The model under review builds one solid part; all positions refer to its coordinate system, in mm. Face numbers are marked on the shaded views. A direction names the side the tool comes from. Round coordinates to 2 decimals unless told otherwise and drop trailing zeros. Order: outer loops, then holes, each group sorted by start corner. A loop starts at its lowest first (then second) coordinate and runs counter-clockwise, first axis right, second up. Notation, with made-up numbers: M 62,9.5 L 112,9.5 A38 ccw 112,48.5 Z; hole C -30,29.5 d5. An arc over 180 degrees is marked long. Answer as a JSON object with one key per item and string values. Group by question number.
1. Add section B-B on z = 23. State the section outline as (x, y) points, and give its area (3 significant figures).
2. To check wall thickness, follow probe 1 along X at (y, z) = (-7.5, 8.25); probe 2 along Z at (x, y) = (15.5, 2); probe 3 along Y at (x, z) = (38, 5). State the ranges of each line that lie inside material, in increasing order. Write a range as [from, to].
3. Add section D-D on z = 5.5. State the section outline as (x, y) points.
4. Clearance check with flat-ended pins moving along their axes: P1, Ø4, axis at x = 23, z = 15.5, coming from the +Y side; P2, Ø1, axis at x = 22.5, z = 8.5, coming from the -Y side; P3, Ø8, axis at x = 26, z = 16, coming from the +Y side. State where each tip first meets the part, or that it passes through.
5. Add section A-A on y = -37. State the section outline as (x, z) points.
6. Mouldability with a two-part tool opening along X and no side actions: class the marked faces 4, 5 and 6 as released by +X, released by -X, zero draft, split by the parting line, or undercut.
7. Add section C-C on y = -13.5. State the section outline as (x, z) points.
8. Machinability: for the marked faces 1, 2 and 3, which of the approach directions +Z, -Z, +X, -X, +Y, -Y give a long, thin tool a straight path to every point of the face, cutting with its end or side? Answer none if there is none.
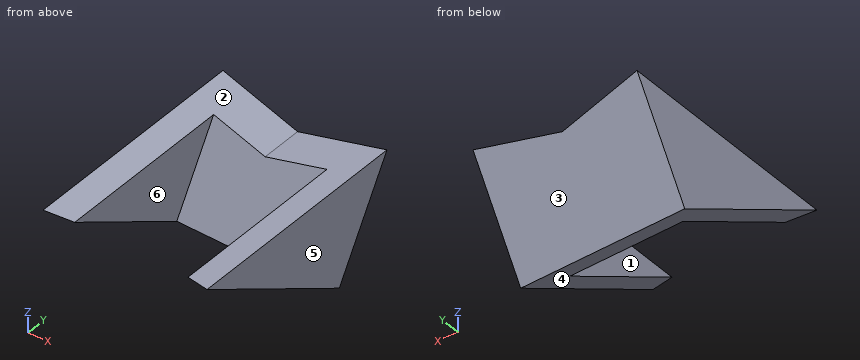
```python
from build123d import *

# Parameters (mm, degrees)
EXTRUDE_1_DEPTH     = 42
CUT_EXTRUDE_3_DEPTH = 77.352761936
SKETCH_4_W          = 29
SKETCH_4_H          = 38.596109301
CUT_EXTRUDE_4_DEPTH = 42


with BuildPart() as part:
    # Эскиз1 → Бобышка-Вытянуть1 (new body)
    with BuildSketch(Plane(origin=(0, 0, 0), x_dir=(0, 0, -1), z_dir=(1, 0, 0))):
        Polygon((0, 0), (-25.751903746, 15.473304826), (-25.751903746, -42.858365035), align=None)
    extrude(amount=EXTRUDE_1_DEPTH)

    # Эскиз3 → Вырез-Вытянуть3 (cut, through all)
    with BuildSketch(Plane(origin=(0, 15.473304826, 0), x_dir=(1, 0, 0), z_dir=(0, 1, 0))):
        Polygon((0, -25.751903746), (21, -21.751903746), (42, -25.751903746), align=None)
    extrude(amount=-CUT_EXTRUDE_3_DEPTH, mode=Mode.SUBTRACT)

    # Эскиз4 → Вырез-Вытянуть4 (cut)
    with BuildSketch(Plane(origin=(0, 0, 0), x_dir=(-1, 0, 0), z_dir=(0, -0.5150380749100486, -0.8571673007021157))):
        with Locations((-21, -28.298054651)):
            Rectangle(SKETCH_4_W, SKETCH_4_H)
    extrude(amount=-CUT_EXTRUDE_4_DEPTH, mode=Mode.SUBTRACT)


solid = part.part
```
Recorded:
{
 "1": {"outline": "M 0,-38.28 L 6.5,-38.28 L 6.5,3.32 L 14.45,3.32 L 14.45,13.82 L 0,13.82 Z; M 27.55,3.32 L 35.5,3.32 L 35.5,-38.28 L 42,-38.28 L 42,13.82 L 27.55,13.82 Z", "area": "844 mm²"},
 "2": {"probe 1": "x = [0, 6.5], [35.5, 42]", "probe 2": "z = [3.33, 20.8]", "probe 3": "y = [-8.32, 3]"},
 "3": {"outline": "M 0,-9.15 L 6.5,-9.15 L 6.5,-7.19 L 35.5,-7.19 L 35.5,-9.15 L 42,-9.15 L 42,3.3 L 0,3.3 Z"},
 "4": {"P1": "stops at y = 10.52", "P2": "stops at y = -5.69", "P3": "stops at y = 12.02"},
 "5": {"outline": "M 0,22.23 L 6.5,22.23 L 6.5,24.51 L 0,25.75 Z; M 35.5,22.23 L 42,22.23 L 42,25.75 L 35.5,24.51 Z"},
 "6": {"face 4": "zero draft", "face 5": "released by +X", "face 6": "undercut"},
 "7": {"outline": "M 0,8.11 L 6.5,8.11 L 6.5,24.51 L 0,25.75 Z; M 35.5,8.11 L 42,8.11 L 42,25.75 L 35.5,24.51 Z"},
 "8": {"face 1": "+Z, -Y", "face 2": "+Z, +Y, -Y", "face 3": "-Z, +X, -X, +Y"}
}
